Verification items for this drawing (mm, ordinates from the low corner). A direction names the side the tool comes from. Give positions to 0.01 mm unless a question says otherwise; leave off trailing zeros. Loops run counter-clockwise (first coordinate to the right, second up) from the corner with the lowest first, then second, coordinate; pieces in that order, holes last. Notation, with made-up numbers: (-18.75, -40) -> (-9.75, -40) arc R31 cw to (-9.75, -1) -> close; hole circle Ø9 at (-20, 27). An arc over 180 degrees is marked (long way). Answer in a Markdown table with one row per item. Add a question column.
Q1. Set-up check for the marked faces 4 and 5: record each of +Z, -Z, +X, -X, +Y, -Y from which the full face is reachable in a straight line by a thin tool's end or side.
Q2. Gauge pin test, flat ends, axial feed: P1, Ø2, axis at x = 7.5, y = 1, coming from the -Z side; P2, Ø3, axis at x = 5, z = 14.5, coming from the +Y side; P3, Ø4, axis at x = 6, y = 3, coming from the +Z side; P4, Ø3, axis at x = 10, z = 7.5, coming from the -Y side. Record the tip position at first contact, or that the pin passes through.
Q3. Section check B-B on y = 4. Enter the section's corners in (x, z).
Q4. Release check for a two-part mould opening along X. For the marked faces 1, 2 and 3 record: pulls with the +X half, pulls with the -X half, needs draft (parallel to the pull), parting line crosses it, or undercut.
Q5. Section check A-A on x = 6. Enter the section's corners in (y, z).
Q6. Material ranges on probe 1 along Z at (x, y) = (8.25, 4); probe 2 along Z at (x, y) = (3.5, 1); probe 3 along Y at (x, z) = (6, 18.5), recorded low to high.
Q7. Section check C-C on z = 14.5. Enter the section's corners in (x, y) (3 decimals).
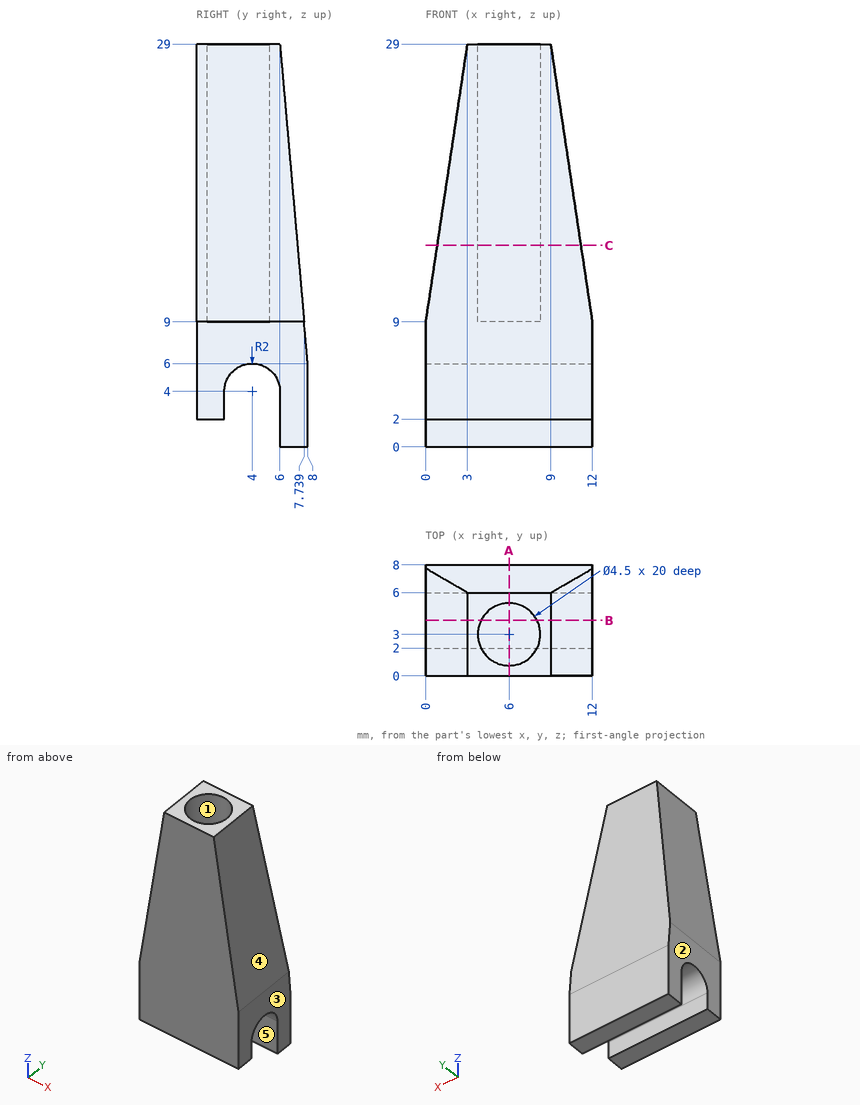
Taken from the geometry:
| question | item | result |
|---|---|---|
| 1 | face 4 | +Z, +X, +Y, -Y |
| 1 | face 5 | -Z, +X, -X |
| 2 | P1 | stops at z = 2 |
| 2 | P2 | stops at y = 7.39 |
| 2 | P3 | stops at z = 9 |
| 2 | P4 | stops at y = 0 |
| 3 | outline | (0, 6) -> (12, 6) -> (12, 9) -> (9, 29) -> (8.02, 29) -> (8.02, 9) -> (3.98, 9) -> (3.98, 29) -> (3, 29) -> (0, 9) -> close |
| 4 | face 1 | undercut |
| 4 | face 2 | pulls with the -X half |
| 4 | face 3 | pulls with the +X half |
| 5 | outline | (0, 2) -> (2, 2) -> (2, 4) arc R2 cw to (6, 4) -> (6, 0) -> (8, 0) -> (8, 6) -> (6, 29) -> (5.25, 29) -> (5.25, 9) -> (0.75, 9) -> (0.75, 29) -> (0, 29) -> close |
| 6 | probe 1 | z = 6 to 29 |
| 6 | probe 2 | z = 2 to 29 |
| 6 | probe 3 | y = 0 to 0.75, 5.25 to 6.91 |
| 7 | outline | (0.825, 0) -> (11.175, 0) -> (11.175, 7.261) -> (0.825, 7.261) -> close; hole circle Ø4.5 at (6, 3) |
